Verification items for the finished model (mm, model axes). Round coordinates to 2 decimals unless told otherwise and drop trailing zeros. Loops run counter-clockwise (first coordinate to the right, second up) from the corner with the lowest first, then second, coordinate; pieces in that order, holes last. Notation, with made-up numbers: (83.25, 86) -> (131.25, 86) arc R20 cw to (131.25, 122) -> close; hole circle Ø1 at (-29, -30). An arc over 180 degrees is marked (long way). Use a Markdown table: item, result. Add a question column.
```python
from build123d import *

# Parameters (mm, degrees)
ESQUISSE1_W        = 80
ESQUISSE1_H        = 47
ESQUISSE1_R        = 2
BOSS_EXTRU_1_DEPTH = 3
CONG_1_R           = 4


with BuildPart() as part:
    # Esquisse1 → Boss.-Extru.1 (new body)
    with BuildSketch(Plane.XY):
        with Locations((40, -23.5)):
            Rectangle(ESQUISSE1_W, ESQUISSE1_H)
        with Locations((5, -4)):
            Circle(ESQUISSE1_R, mode=Mode.SUBTRACT)
        with Locations((75, -4)):
            Circle(ESQUISSE1_R, mode=Mode.SUBTRACT)
    extrude(amount=BOSS_EXTRU_1_DEPTH)

    # Congé1
    cong_1_edges = [part.edges().sort_by_distance(p)[0] for p in [
        (0, 0, 1.5),
        (80, 0, 1.5),
        (80, -47, 1.5),
        (0, -47, 1.5),
    ]]
    fillet(cong_1_edges, radius=CONG_1_R)


solid = part.part
```
1) Thickness scan on line 1 (Y direction, x = 5, z = 1.25); line 2 (X direction, y = -45, z = 2.65). Record the ranges inside material, lowest first.
2) Sectioned sample at A-A on x = 75. Enter the section's corners in (y, z).
3) Release check for a two-part mould opening along Z. For faces 1 (the face through (39, -23, 3)), 2 (the face through (39, -23, 0)), 3 (the face through (1.141, -45.797, 1.521)) record: released by +Z, released by -Z, zero draft, split by the parting line, or undercut.
Geometry results:
| question | item | result |
|---|---|---|
| 1 | line 1 | -47 to -6, -2 to 0 |
| 1 | line 2 | 0.54 to 79.46 |
| 2 | outline | (-47, 0) -> (-6, 0) -> (-6, 3) -> (-47, 3) -> close; (-2, 0) -> (0, 0) -> (0, 3) -> (-2, 3) -> close |
| 3 | face 1 | released by +Z |
| 3 | face 2 | released by -Z |
| 3 | face 3 | zero draft |
